The listing builds one solid part. Answer for the finished solid, in the listing's coordinates (mm). Round coordinates to 2 decimals unless told otherwise and drop trailing zeros. Order: outer loops, then holes, each group sorted by start corner. A loop starts at its lowest first (then second) coordinate and runs counter-clockwise, first axis right, second up. Notation, with made-up numbers: (16.25, 79.5) -> (37.25, 79.5) arc R24 ccw to (37.25, 114.5) -> close; hole circle Ø5 at (74, 68). An arc over 180 degrees is marked (long way). Answer in a Markdown table with one row per item. Add a question column.
Autodesk Inventor part; units mm, degrees
ref_plane "YZ Plane" through (0, 0, 0) normal (1, 0, 0) x (0, 1, 0)
ref_plane "XZ Plane" through (0, 0, 0) normal (0, 1, 0) x (-1, 0, 0)
ref_plane "XY Plane" through (0, 0, 0) normal (0, 0, 1) x (1, 0, 0)
sketch "Sketch1" plane through (0, 0, 0) normal (0, 0, 1) x (1, 0, 0)
  line L0 (0, 10) -> (0, 37.7157)
  line L1 (5.8579, 51.8579) -> (27.0711, 73.0711)
  line L2 (34.1421, 76) -> (45.8579, 76)
  line L3 (52.9289, 73.0711) -> (74.1421, 51.8579)
  line L4 (80, 37.7157) -> (80, 10)
  line L5 (70, 0) -> (10, 0)
  circle A0 centre (12.5, 12.5) radius 1.675
  circle A1 centre (67.5, 12.5) radius 1.675
  circle A2 centre (67.5, 33.5) radius 2
  circle A3 centre (12.5, 33.5) radius 2
  circle A4 centre (40, 12.5) radius 2
  circle A5 centre (40, 33.5) radius 2
  circle A6 centre (40, 62) radius 10
  arc A7 (5.8579, 51.8579) -> (0, 37.7157) centre (20, 37.7157) ccw
  arc A8 (0, 10) -> (10, 0) centre (10, 10) ccw
  arc A9 (70, 0) -> (80, 10) centre (70, 10) ccw
  arc A10 (80, 37.7157) -> (74.1421, 51.8579) centre (60, 37.7157) ccw
  arc A11 (34.1421, 76) -> (27.0711, 73.0711) centre (34.1421, 66) ccw
  arc A12 (52.9289, 73.0711) -> (45.8579, 76) centre (45.8579, 66) ccw
  point P0 (0, 0)
  point P1 (0, 46)
  point P2 (30, 76)
  point P3 (50, 76)
  point P4 (80, 46)
  point P5 (80, 0)
  point P6 (40, 0)
  point P7 (40, 76)
  dimension "d0" = 46
  dimension "d1" = 46
  dimension "d2" = 80
  dimension "d3" = 30
  dimension "d4" = 30
  dimension "d5" = 30
  dimension "d6" = 3.35
  dimension "d10" = 3.35
  dimension "d12" = 12.5
  dimension "d13" = 12.5
  dimension "d14" = 12.5
  dimension "d15" = 12.5
  dimension "d16" = 4
  dimension "d18" = 12.5
  dimension "d19" = 12.5
  dimension "d20" = 4
  dimension "d22" = 12.5
  dimension "d23" = 12.5
  dimension "d25" = 4
  dimension "d27" = 12.5
  dimension "d28" = 4
  dimension "d30" = 20
  dimension "d31" = 14
  dimension "d32" = 20
  dimension "d33" = 40
  dimension "d34" = 40
  dimension "d35" = 10
  dimension "d36" = 10
  dimension "d37" = 20
  dimension "d38" = 10
  dimension "d39" = 10
extrude "Plate1" add sketch "Sketch1" along normal blind 1.5
equation "\"d6\" = rivet_diameter"
equation "\"d10\" = rivet_diameter"
equation "\"d12\" = rivet_wall_clearance"
equation "\"d14\" = rivet_wall_clearance"
equation "\"d15\" = rivet_wall_clearance"
equation "\"d16\" = d17"
equation "\"d18\" = rivet_wall_clearance"
equation "\"d20\" = d21"
equation "\"d23\" = rivet_wall_clearance"
equation "\"d25\" = d26"
equation "\"d27\" = rivet_wall_clearance"
equation "\"d28\" = d29"
equation "\"d24\" = Thickness"
equation "\"BendRadius\" = Thickness"
equation "\"BendReliefWidth\" = Thickness"
equation "\"BendReliefDepth\" = 0.5 * Thickness"
equation "\"CornerReliefSize\" = 4 * Thickness"
equation "\"MinimumRemnant\" = 2 * Thickness"
equation "\"TransitionRadius\" = BendRadius"
equation "\"JacobiRadiusSize\" = BendRadius"
equation "\"GapSize\" = Thickness"
equation "\"A_width\" = 46"
equation "\"A_joint_diameter\" = 16"
equation "\"A_joint_tolerance\" = 3"
equation "\"l___________\" = 0"
equation "\"l__________\" = 0"
equation "\"l_________\" = 0"
equation "\"rivet_diameter\" = 3.35"
equation "\"plate_thickness\" = 3"
equation "\"l________\" = 0"
equation "\"L_Piston_Top\" = 25"
equation "\"L_Piston_Bottom\" = 21"
equation "\"rivet_wall_clearance\" = 12.5"
equation "\"thin_plate\" = 1.5"
equation "\"A_B_spacing\" = 2"
properties part number "sideplate"
1. The part is cut by section D-D (y = 62). Give the vertices of the cut face in (x, z).
2. The part is cut by section B-B (y = 33.5). Give the vertices of the cut face in (x, z).
3. The part is cut by section A-A (x = 40). Give the vertices of the cut face in (y, z), then the cut area to 3 significant figures.
4. Straight lines are drawn through the part: line 1 along Y through (x, z) = (40, 0.55); line 2 along X through (y, z) = (35, 1.45); line 3 along X through (y, z) = (13, 0.85). For each, find the intervals that lie inside material, in ascending order.
5. The part is cut by section C-C (x = 12.5). Give the vertices of the cut face in (y, z) (3 decimals).
6. The mould has two halves that part along Y. Classify faces 1 (the flat face through (39, 30, 0)), 2 (the cylindrical face through (77.15, 3.01, 0.74)), 3 (the cylindrical face through (78.435, 45.471, 0.74)), 4 (the cylindrical face through (37.83, 71.76, 0.74)): released by +Y, released by -Y, zero draft, split by the parting line, or undercut.
Report:
| question | item | result |
|---|---|---|
| 1 | outline | (16, 0) -> (30, 0) -> (30, 1.5) -> (16, 1.5) -> close; (50, 0) -> (64, 0) -> (64, 1.5) -> (50, 1.5) -> close |
| 2 | outline | (0, 0) -> (10.5, 0) -> (10.5, 1.5) -> (0, 1.5) -> close; (14.5, 0) -> (38, 0) -> (38, 1.5) -> (14.5, 1.5) -> close; (42, 0) -> (65.5, 0) -> (65.5, 1.5) -> (42, 1.5) -> close; (69.5, 0) -> (80, 0) -> (80, 1.5) -> (69.5, 1.5) -> close |
| 3 | outline | (0, 0) -> (10.5, 0) -> (10.5, 1.5) -> (0, 1.5) -> close; (14.5, 0) -> (31.5, 0) -> (31.5, 1.5) -> (14.5, 1.5) -> close; (35.5, 0) -> (52, 0) -> (52, 1.5) -> (35.5, 1.5) -> close; (72, 0) -> (76, 0) -> (76, 1.5) -> (72, 1.5) -> close |
| 3 | area | 72.0 mm^2 |
| 4 | line 1 | y = 0 to 10.5, 14.5 to 31.5, 35.5 to 52, 72 to 76 |
| 4 | line 2 | x = 0 to 11.18, 13.82 to 38.68, 41.32 to 66.18, 68.82 to 80 |
| 4 | line 3 | x = 0 to 10.9, 14.1 to 38.06, 41.94 to 65.9, 69.1 to 80 |
| 5 | outline | (0, 0) -> (10.825, 0) -> (10.825, 1.5) -> (0, 1.5) -> close; (14.175, 0) -> (31.5, 0) -> (31.5, 1.5) -> (14.175, 1.5) -> close; (35.5, 0) -> (58.5, 0) -> (58.5, 1.5) -> (35.5, 1.5) -> close |
| 6 | face 1 | zero draft |
| 6 | face 2 | released by -Y |
| 6 | face 3 | released by +Y |
| 6 | face 4 | undercut |
